from build123d import *

# Parameters (mm, degrees)
SKETCH2_W           = 54.022158158
SKETCH2_H           = 36.022158158
SKETCH2_W_2         = 46.5
SKETCH2_H_2         = 28.5
BOSS_EXTRUDE1_DEPTH = 34.036
SKETCH3_W           = 8.658958029
SKETCH3_H           = 53.977841842
SKETCH3_W_2         = 35.977841842
SKETCH3_H_2         = 8.658958029
BOSS_EXTRUDE2_DEPTH = 30
BOSS_EXTRUDE3_DEPTH = 6.35
SKETCH5_W           = 20
SKETCH5_H           = 6.78
SKETCH5_W_2         = 6.78
SKETCH5_H_2         = 20
BOSS_EXTRUDE4_DEPTH = 10
FILLET1_R           = 2.54
SKETCH11_R          = 1.049999932
CUT_EXTRUDE1_DEPTH  = 132.751467908


with BuildPart() as part:
    # Sketch2 → Boss-Extrude1 (new body)
    with BuildSketch(Plane(origin=(0, 0, 0), x_dir=(1, 0, 0), z_dir=(0, 1, 0))):
        with Locations((27.011079079, -18.011079079)):
            Rectangle(SKETCH2_W, SKETCH2_H)
        with Locations((27.011079079, -18.011079079)):
            Rectangle(SKETCH2_W_2, SKETCH2_H_2, mode=Mode.SUBTRACT)
    extrude(amount=-BOSS_EXTRUDE1_DEPTH)

    # Sketch3 → Boss-Extrude2 (add)
    with BuildSketch(Plane(origin=(0, 0, 0), x_dir=(1, 0, 0), z_dir=(0, 1, 0))):
        with Locations((4.329479015, -63.011079079)):
            Rectangle(SKETCH3_W, SKETCH3_H)
        with Locations((72.011079079, -4.329479015)):
            Rectangle(SKETCH3_W_2, SKETCH3_H_2)
    extrude(amount=-BOSS_EXTRUDE2_DEPTH)

    # Sketch4 → Boss-Extrude3 (add)
    with BuildSketch(Plane(origin=(0, 0, 0), x_dir=(1, 0, 0), z_dir=(0, 1, 0))):
        Polygon((0, -90), (8.658958029, -90), (8.658958029, -70), (0, -70), (-10, -70), (-16.78, -70), (-16.78, -90), (-10, -90), align=None)
        Polygon((90, -8.658958029), (90, 0), (90, 10), (90, 16.78), (70, 16.78), (70, 10), (70, 0), (70, -8.658958029), align=None)
    extrude(amount=BOSS_EXTRUDE3_DEPTH)

    # Sketch5 → Boss-Extrude4 (add)
    with BuildSketch(Plane.XZ):
        with Locations((80, -13.39)):
            Rectangle(SKETCH5_W, SKETCH5_H)
        with Locations((-13.39, 80)):
            Rectangle(SKETCH5_W_2, SKETCH5_H_2)
    extrude(amount=BOSS_EXTRUDE4_DEPTH)

    # Fillet1
    fillet1_edges = [part.edges().sort_by_distance(p)[0] for p in [
        (80, -10, -16.78),
        (-16.78, -1.825, 70),
        (-16.78, -1.825, 90),
        (-4.060520985, 6.35, 90),
        (8.658958029, 6.35, 80),
        (-4.060520985, 6.35, 70),
        (-16.78, 6.35, 80),
        (90, -1.825, -16.78),
        (70, -1.825, -16.78),
        (80, 6.35, 8.658958029),
        (90, 6.35, -4.060520985),
        (80, 6.35, -16.78),
        (70, 6.35, -4.060520985),
        (-16.78, -10, 80),
    ]]
    fillet(fillet1_edges, radius=FILLET1_R)

    # Sketch11 → Cut-Extrude1 (cut, through all)
    with BuildSketch(Plane(origin=(0, 0, 0), x_dir=(-1, 0, 0), z_dir=(0, 0, -1))):
        with Locations((-19.011079079, -11)):
            Circle(SKETCH11_R)
        with Locations((-19.011079079, -23)):
            Circle(SKETCH11_R)
        with Locations((-43.01107908, -11)):
            Circle(SKETCH11_R)
        with Locations((-43.011079079, -23)):
            Circle(SKETCH11_R)
    extrude(amount=-CUT_EXTRUDE1_DEPTH, mode=Mode.SUBTRACT)


solid = part.part
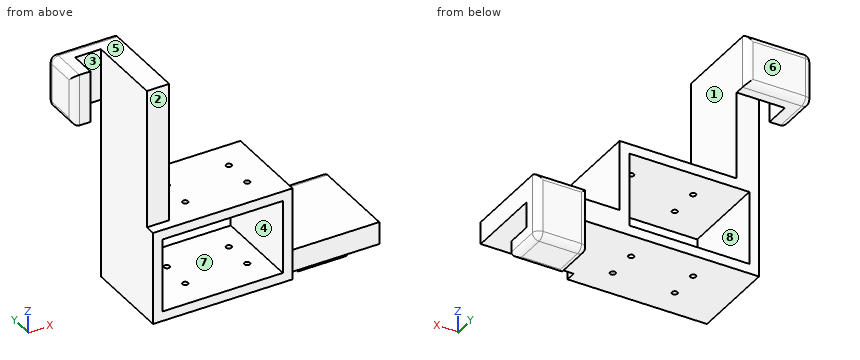
The listing builds one solid part. Answer for the finished solid, in the listing's coordinates (mm). Face numbers are marked on the shaded views. A direction names the side the tool comes from. Coordinates: 2 decimals unless noted, no trailing zeros. Write each loop counter-clockwise with the first axis right and the second up, starting at its lowest first coordinate (ties: lowest second). Pieces come first, ordered by that corner, then holes. Notation, with made-up numbers: M 60,-22 L 117,-22 A20 ccw 117,4 Z; hole C 44,-26.75 d5. An arc over 180 degrees is marked long. Use one line per item in the form item = value.
Item 1: Find section B-B, the plane z = 30. Give the vertices of the cut face in (x, y).
Model answer:
outline = M 0,-34.04 L 3.76,-34.04 L 3.76,0 L 0,0 Z; M 50.26,-34.04 L 54.02,-34.04 L 54.02,0 L 50.26,0 Z
Item 2: Given P1, Ø17, axis at x = 23, y = -24, coming from the +Z side; P2, Ø2.5, axis at x = 2.5, z = 68.5, coming from the -Y side; P3, Ø3.5, axis at x = 43.01, y = -23, coming from the -Z side; P4, Ø1.9, axis at x = 19.01, y = -23, coming from the -Z side, each flat-ended and moving along its own axis, determine where each tip first touches the part or whether it passes through.
Model answer:
P1 = 36.02
P2 = -30
P3 = 0
P4 = through
Item 3: Find the intervals of material crossed by probe 1 along Z at (x, y) = (14.5, -8); probe 2 along X at (y, z) = (-19, 15); probe 3 along X at (y, z) = (-18, 6), in increasing order.
Model answer:
probe_1 = 0 to 3.76, 32.26 to 36.02
probe_2 = 0 to 3.76, 50.26 to 54.02
probe_3 = 0 to 3.76, 50.26 to 90
Item 4: Find section D-D, the plane y = -19. Give the vertices of the cut face in (x, z), plus the area to 3 significant figures.
Model answer:
outline = M 0,0 L 90,0 L 90,8.66 L 54.02,8.66 L 54.02,36.02 L 8.66,36.02 L 8.66,90 L 0,90 Z; hole M 3.76,3.76 L 50.26,3.76 L 50.26,32.26 L 3.76,32.26 Z
area = 1,400 mm2
Item 5: Find section A-A, the plane y = -5.5. Give the vertices of the cut face in (x, z), plus the area to 3 significant figures.
Model answer:
outline = M -16.78,72.54 A2.54 ccw -14.24,70 L -10,70 L -10,90 L -14.24,90 A2.54 ccw -16.78,87.46 Z; M 0,0 L 90,0 L 90,8.66 L 54.02,8.66 L 54.02,36.02 L 8.66,36.02 L 8.66,90 L 0,90 Z; M 70,-14.24 A2.54 ccw 72.54,-16.78 L 87.46,-16.78 A2.54 ccw 90,-14.24 L 90,-10 L 70,-10 Z; hole M 3.76,3.76 L 50.26,3.76 L 50.26,32.26 L 3.76,32.26 Z
area = 1,670 mm2
Item 6: The mould has two halves that part along Z. Classify the marked faces 5, 6, 7 and 8: released by +Z, released by -Z, zero draft, split by the parting line, or undercut.
Model answer:
face_5 = released by +Z
face_6 = zero draft
face_7 = undercut
face_8 = undercut
Item 7: For the marked faces 1, 2, 3 and 4, determine the directions among +Z, -Z, +X, -X, +Y, -Y from which every point of the face is accessible in a straight line to the end or side of a thin tool.
Model answer:
face_1 = +Z, +X, +Y, -Y
face_2 = +Z, +X, -X, -Y
face_3 = +Z, -Z, -Y
face_4 = +Y, -Y
Item 8: Find section C-C, the plane x = 10.5. Give the vertices of the cut face in (y, z), plus the area to 3 significant figures.
Model answer:
outline = M -34.04,0 L 0,0 L 0,3.76 L -34.04,3.76 Z; M -34.04,32.26 L 0,32.26 L 0,36.02 L -34.04,36.02 Z
area = 256 mm2
